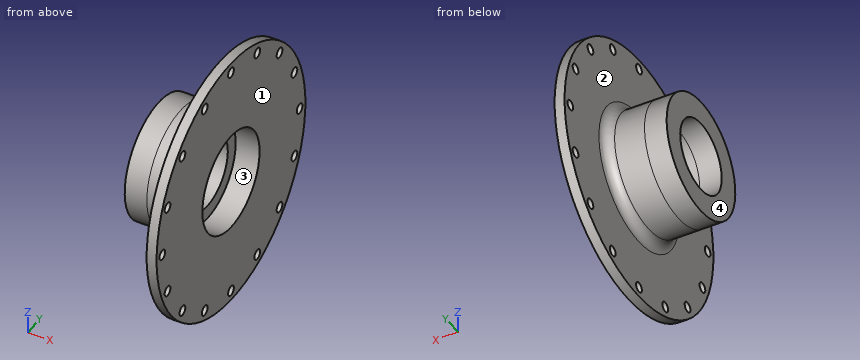
```python
from build123d import *

# Parameters (mm, degrees)
SKETCH1_R           = 130
SKETCH1_R_2         = 5
SKETCH1_R_3         = 36.2419
BOSS_EXTRUDE1_DEPTH = 10
BOSS_EXTRUDE2_START = -50
SKETCH2_R           = 60
SKETCH2_R_2         = 36.2419
BOSS_EXTRUDE2_DEPTH = 50
FILLET1_R           = 10
SKETCH3_R           = 50
CUT_EXTRUDE1_DEPTH  = 24
BOSS_EXTRUDE3_START = 22.2
SKETCH4_R           = 60
SKETCH4_R_2         = 36.2419
BOSS_EXTRUDE3_DEPTH = 22.2


with BuildPart() as part:
    # Sketch1 → Boss-Extrude1 (new body)
    with BuildSketch(Plane(origin=(0, 0, 0), x_dir=(0, 0, -1), z_dir=(1, 0, 0))):
        Circle(SKETCH1_R)
        with Locations((0, 120)):
            Circle(SKETCH1_R_2, mode=Mode.SUBTRACT)
        with Locations((45.922011884, 110.865543901)):
            Circle(SKETCH1_R_2, mode=Mode.SUBTRACT)
        with Locations((84.852813742, 84.852813742)):
            Circle(SKETCH1_R_2, mode=Mode.SUBTRACT)
        with Locations((110.865543901, 45.922011884)):
            Circle(SKETCH1_R_2, mode=Mode.SUBTRACT)
        with Locations((120, 0)):
            Circle(SKETCH1_R_2, mode=Mode.SUBTRACT)
        with Locations((110.865543901, -45.922011884)):
            Circle(SKETCH1_R_2, mode=Mode.SUBTRACT)
        with Locations((84.852813742, -84.852813742)):
            Circle(SKETCH1_R_2, mode=Mode.SUBTRACT)
        with Locations((45.922011884, -110.865543901)):
            Circle(SKETCH1_R_2, mode=Mode.SUBTRACT)
        with Locations((0, -120)):
            Circle(SKETCH1_R_2, mode=Mode.SUBTRACT)
        with Locations((-45.922011884, -110.865543901)):
            Circle(SKETCH1_R_2, mode=Mode.SUBTRACT)
        with Locations((-84.852813742, -84.852813742)):
            Circle(SKETCH1_R_2, mode=Mode.SUBTRACT)
        with Locations((-110.865543901, -45.922011884)):
            Circle(SKETCH1_R_2, mode=Mode.SUBTRACT)
        with Locations((-120, 0)):
            Circle(SKETCH1_R_2, mode=Mode.SUBTRACT)
        with Locations((-110.865543901, 45.922011884)):
            Circle(SKETCH1_R_2, mode=Mode.SUBTRACT)
        with Locations((-84.852813742, 84.852813742)):
            Circle(SKETCH1_R_2, mode=Mode.SUBTRACT)
        with Locations((-45.922011884, 110.865543901)):
            Circle(SKETCH1_R_2, mode=Mode.SUBTRACT)
        Circle(SKETCH1_R_3, mode=Mode.SUBTRACT)
    extrude(amount=BOSS_EXTRUDE1_DEPTH)

    # Sketch2 → Boss-Extrude2 (add)
    with BuildSketch(Plane(origin=(10, 0, 0), x_dir=(0, 0, -1), z_dir=(1, 0, 0)).offset(BOSS_EXTRUDE2_START)):
        Circle(SKETCH2_R)
        Circle(SKETCH2_R_2, mode=Mode.SUBTRACT)
    extrude(amount=BOSS_EXTRUDE2_DEPTH)

    # Fillet1
    fillet1_edges = [part.edges().sort_by_distance(p)[0] for p in [
        (0, 0, 60),
    ]]
    fillet(fillet1_edges, radius=FILLET1_R)

    # Sketch3 → Cut-Extrude1 (cut)
    with BuildSketch(Plane(origin=(10, 0, 0), x_dir=(0, 0, -1), z_dir=(1, 0, 0))):
        Circle(SKETCH3_R)
    extrude(amount=-CUT_EXTRUDE1_DEPTH, mode=Mode.SUBTRACT)

    # Sketch4 → Boss-Extrude3 (add)
    with BuildSketch(Plane.ZY.offset(40).offset(BOSS_EXTRUDE3_START)):
        with Locations(Location((0, 0, 0), (0, 0, 180))):
            Circle(SKETCH4_R)
        Circle(SKETCH4_R_2, mode=Mode.SUBTRACT)
    extrude(amount=-BOSS_EXTRUDE3_DEPTH)


solid = part.part
```
Source: CAD feature listing. Evaluate the final solid. Frame: model axes, mm. Face numbers are marked on the shaded views. A direction names the side the tool comes from. Coordinates: 2 decimals unless noted, no trailing zeros. Write each loop counter-clockwise with the first axis right and the second up, starting at its lowest first coordinate (ties: lowest second). Pieces come first, ordered by that corner, then holes. Notation, with made-up numbers: (38.5, -18.5) -> (84.5, -18.5) arc R8 cw to (84.5, -7.5) -> close; hole circle Ø11 at (-4.5, 63.25). An arc over 180 degrees is marked (long way). Return JSON: item names as keys, results as strings. Group by question number.
1) Ray query, line 1 along Y through (x, z) = (5, 0); line 2 along Y through (x, z) = (6, -120); line 3 along Z through (x, y) = (-30.5, 0). Return the intervals inside material, ascending.
2) Section query C-C, the plane y = 0. Return loops of the section in (x, z).
3) Section query A-A, the plane z = -120. Return loops of the section in (x, y).
4) Section query D-D, the plane z = 84.5. Return loops of the section in (x, y).
5) Contact query for flat-ended pins moving along their axis: P1, Ø13, axis at y = -120, z = 0, coming from the -X side; P2, Ø2, axis at x = -22, y = -26, coming from the +Z side; P3, Ø8, axis at x = -20, y = 57.5, coming from the -Z side; P4, Ø16, axis at y = -84.85, z = 84.85, coming from the +X side. Output: stop coordinate, or through.
6) Set-up query: the marked faces 1 and 2. Return all of +Z, -Z, +X, -X, +Y, -Y with unobstructed straight access to the full face (end or side cutting, diameter ignored); none if empty.
7) Mould query, pull axis Y, two halves, no side actions, for the marked faces 3 and 4. Classes: +Y half, -Y half, draft (parallel to the pull), parting line (faces both ways), or undercut.
From the geometry:
{
 "1": {"line 1": "-130 to -125, -115 to -50, 50 to 115, 125 to 130", "line 2": "-50 to -5, 5 to 50", "line 3": "-60 to -36.24, 36.24 to 60"},
 "2": {"outline": "(-62.2, -60) -> (-10, -60) arc R10 cw to (0, -70) -> (0, -115) -> (10, -115) -> (10, -50) -> (-14, -50) -> (-14, -36.24) -> (-62.2, -36.24) -> close; (-62.2, 36.24) -> (-14, 36.24) -> (-14, 50) -> (10, 50) -> (10, 115) -> (0, 115) -> (0, 70) arc R10 cw to (-10, 60) -> (-62.2, 60) -> close; (0, -130) -> (10, -130) -> (10, -125) -> (0, -125) -> close; (0, 125) -> (10, 125) -> (10, 130) -> (0, 130) -> close"},
 "3": {"outline": "(0, -50) -> (10, -50) -> (10, -5) -> (0, -5) -> close; (0, 5) -> (10, 5) -> (10, 50) -> (0, 50) -> close"},
 "4": {"outline": "(0, -98.79) -> (10, -98.79) -> (10, -89.84) -> (0, -89.84) -> close; (0, -79.87) -> (10, -79.87) -> (10, 79.87) -> (0, 79.87) -> close; (0, 89.84) -> (10, 89.84) -> (10, 98.79) -> (0, 98.79) -> close"},
 "5": {"P1": "x = 0", "P2": "z = 54.54", "P3": "z = -27.16", "P4": "x = 10"},
 "6": {"face 1": "+Z, -Z, +X, +Y, -Y", "face 2": "-X"},
 "7": {"face 3": "undercut", "face 4": "draft"}
}
